Could you check a few things on this model? Use its own coordinates, in mm. A direction names the side the tool comes from. Coordinates: 2 decimals unless noted, no trailing zeros. One line per question, with ' | ' between items. Start each with the question number.
from build123d import *

# Parameters (mm, degrees)
CROQUIS1_R                                           = 55.5
SALIENTE_EXTRUIR1_DEPTH                              = 44
CROQUIS2_R                                           = 50.5
CROQUIS2_R_2                                         = 24.75
CORTAR_EXTRUIR2_DEPTH                                = 6.93
REFRENTADO_PARA_TORNILLO_CON_CABEZA_TRON_D           = 9
REFRENTADO_PARA_TORNILLO_CON_CABEZA_TRON_CBORE_D     = 18
REFRENTADO_PARA_TORNILLO_CON_CABEZA_TRON_CBORE_DEPTH = 30
TALADRO_ROSCADO_M10X1_51_D                           = 8.5


with BuildPart() as part:
    # Croquis1 → Saliente-Extruir1 (new body)
    with BuildSketch(Plane(origin=(0, 0, 0), x_dir=(1, 0, 0), z_dir=(0, 1, 0))):
        with Locations(Location((0, 0, 0), (0, 0, 270))):
            Circle(CROQUIS1_R)
    extrude(amount=SALIENTE_EXTRUIR1_DEPTH)

    # Croquis2 → Cortar-Extruir2 (cut)
    with BuildSketch(Plane(origin=(0, 44, 0), x_dir=(1, 0, 0), z_dir=(0, 1, 0))):
        with Locations(Location((0, 0, 0), (0, 0, 270))):
            Circle(CROQUIS2_R)
        with Locations(Location((0, 0, 0), (0, 0, 270))):
            Circle(CROQUIS2_R_2, mode=Mode.SUBTRACT)
    extrude(amount=-CORTAR_EXTRUIR2_DEPTH, mode=Mode.SUBTRACT)

    # Refrentado para tornillo con cabeza troncocónica de M81 (through all)
    with Locations(Plane(origin=(0, 0, 0), x_dir=(-1, 0, 0), z_dir=(0, -1, 0))):
        with Locations((8.40999002, -39.10590835), (-12.269689172, -38.071705079), (-29.661715059, -26.836219178), (-38.071705079, 12.269689172), (-26.836219178, 29.661715059), (-8.40999002, 39.10590835), (29.661715059, 26.836219178), (39.10590835, 8.40999002), (38.071705079, -12.269689172)):
            CounterBoreHole(REFRENTADO_PARA_TORNILLO_CON_CABEZA_TRON_D / 2, REFRENTADO_PARA_TORNILLO_CON_CABEZA_TRON_CBORE_D / 2, REFRENTADO_PARA_TORNILLO_CON_CABEZA_TRON_CBORE_DEPTH)

    # Taladro roscado M10x1.51 (through all)
    with Locations(Plane(origin=(0, 0, 0), x_dir=(-1, 0, 0), z_dir=(0, -1, 0))):
        with Locations((26.755142579, -30.284161629), (-39.604424593, -8.02855234), (12.849282014, 38.31271397)):
            Hole(TALADRO_ROSCADO_M10X1_51_D / 2)


solid = part.part
(1) If I drill on line 1 along X through (y, z) = (20.5, 32); line 2 along X through (y, z) = (37, 38); line 3 along Z through (x, y) = (-9, 27.5), over which ranges is the centre line in solid material (lowest first)? Write a range as from..to.
(2) On a 3-axis mill with a long thin cutter (end or side, diameter ignored), from which of +Z, -Z, +X, -X, +Y, -Y can I reach the whole of each face in a straight line? I mean faces 4 (the flat face through (-22, 37.07, -12)), 5 (the cylindrical face through (-22.52, 14.79, -21.36)), 6 (the cylindrical face through (-42.423, 33.584, -11.451)). Say none if no direction works.
(3) For P1, Ø6, axis at y = 35, z = 8, coming from the -X side; P2, Ø6, axis at y = 35.5, z = -4.5, coming from the -X side; P3, Ø11.5, axis at x = -8.41, z = 39.11, coming from the -Y side; P4, Ø5.5, axis at x = 38.07, z = -12.27, coming from the -Y side, each with a flat end and sliding along its axis, tell me the tip position at first contact or that it passes through.
(4) Imagine slicing it at A-A, the plane y = 24. Count the separate pieces of the cut face and the enclosed holes in it, plus the area to 3 significant figures.
(5) We'd pull the mould along X, two halves only. Please class faces 1 (the flat face through (-41, 30, -13)), 2 (the flat face through (-49, 44, -13)), 3 (the cylindrical face through (-27.31, 18.79, 26.07)): +X half, -X half, draft (parallel to the pull), parting line (faces both ways), or undercut.
Answers:
1) line 1: -45.35..-30.64, -22.87..-13.93, -2.89..5.63, 18.91..22.29, 37.03..45.35 | line 2: -40.45..-12.77, -4.05..7.77, 16.77..40.45 | line 3: -54.77..-40.11, -36.51..30.13, 48.09..54.77
2) face 4: +Y | face 5: -Y | face 6: +Y, -Y
3) P1: x = -55.27 | P2: x = -55.48 | P3: y = 30 | P4: through
4) separate pieces: 1 | enclosed holes: 12 | area: 7,220 mm²
5) face 1: undercut | face 2: draft | face 3: undercut
